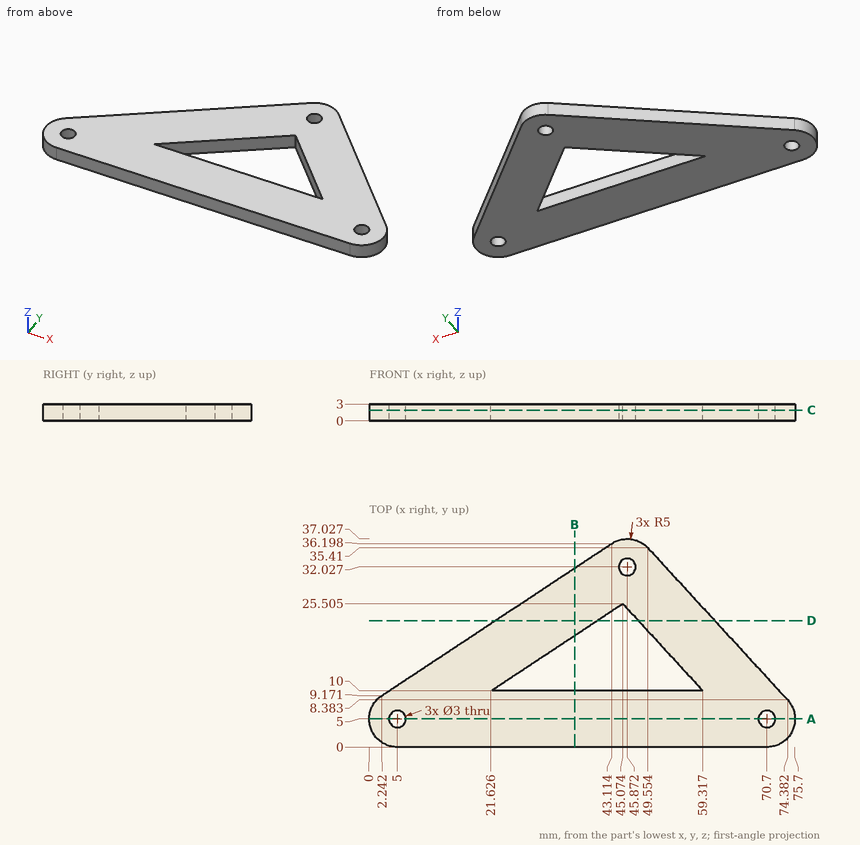
Here's the drawing with two shaded views (mm, measured from the low corner). I have some questions. Give positions to 0.01 mm unless a question says otherwise; leave off trailing zeros. Loops run counter-clockwise (first coordinate to the right, second up) from the corner with the lowest first, then second, coordinate; pieces in that order, holes last. Notation, with made-up numbers: (-37.5, -24.5) -> (-3.5, -24.5) arc R16 cw to (-3.5, -2.5) -> close; hole circle Ø4 at (-15.5, 89). An arc over 180 degrees is marked (long way). One line per item, written item: value.
Q1. Suppose I cut it at B-B on x = 36.5. Please give me the cut outline in (y, z) (1 decimal).
Answers follow:
outline: (0, 0) -> (10, 0) -> (10, 3) -> (0, 3) -> close; (19.8, 0) -> (31.8, 0) -> (31.8, 3) -> (19.8, 3) -> close
Q2. If I drill on line 1 along X through (y, z) = (6, 2.5); line 2 along Y through (x, z) = (44.5, 0.9) (1 decimal); line 3 along X through (y, z) = (32, 1.5) (1 decimal), over which ranges is the centre line in solid material (lowest first)?
Answers follow:
line 1: 0.1 to 3.88, 6.12 to 69.58, 71.82 to 75.6
line 2: 0 to 10, 25.1 to 31.4, 32.6 to 36.8
line 3: 36.8 to 44.4, 47.4 to 52.7
Q3. Suppose I cut it at D-D on y = 22.5. Please give me the cut outline in (x, z) (1 decimal).
Answers follow:
outline: (22.4, 0) -> (40.5, 0) -> (40.5, 3) -> (22.4, 3) -> close; (47.8, 0) -> (61.4, 0) -> (61.4, 3) -> (47.8, 3) -> close
Q4. I'm going to push flat-ended pins straight in: pin 1 Ø3.5 at (x, y) = (5, 5) entering from +Z; pin 2 Ø1.8 at (x, y) = (45.87, 32.03) entering from +Z; pin 3 Ø0.9 at (x, z) = (36.5, 1.5) entering from +Y. Where does each tip first touch, or does it pass through?
Answers follow:
pin 1: z = 3
pin 2: through
pin 3: y = 32.12
Q5. Suppose I cut it at C-C on z = 1.9. Please give me the cut outline in (x, y) (1 decimal).
Answers follow:
outline: (2.2, 9.2) arc R5 ccw to (5, 0) -> (70.7, 0) arc R5 ccw to (74.4, 8.4) -> (49.6, 35.4) arc R5 ccw to (43.1, 36.2) -> close; hole circle Ø3 at (5, 5); hole (21.6, 10) -> (59.3, 10) -> (45.1, 25.5) -> close; hole circle Ø3 at (45.9, 32); hole circle Ø3 at (70.7, 5)
Q6. Suppose I cut it at A-A on y = 5. Please give me the cut outline in (x, z), then the cut area to 3 significant figures.
Answers follow:
outline: (0, 0) -> (3.5, 0) -> (3.5, 3) -> (0, 3) -> close; (6.5, 0) -> (69.2, 0) -> (69.2, 3) -> (6.5, 3) -> close; (72.2, 0) -> (75.7, 0) -> (75.7, 3) -> (72.2, 3) -> close
area: 209 mm^2
